from build123d import *

# Parameters (mm, degrees)
SKETCH1_W           = 4.6
SKETCH1_H           = 2.55
BOSS_EXTRUDE1_DEPTH = 4.6
SKETCH2_W           = 7.97
SKETCH2_H           = 2.55
BOSS_EXTRUDE2_DEPTH = 6.22
SKETCH3_W           = 4.6
SKETCH3_H           = 0.85
BOSS_EXTRUDE3_DEPTH = 0.17
SKETCH4_W           = 4.8
SKETCH4_H           = 2.55
CUT_EXTRUDE1_DEPTH  = 1.29
SKETCH5_W           = 6.77
SKETCH5_H           = 1.15
CUT_EXTRUDE2_DEPTH  = 5.3
CUT_EXTRUDE3_REACH  = 4.55
SKETCH7_W           = 1
SKETCH7_H           = 0.35
BOSS_EXTRUDE4_DEPTH = 3.3
SKETCH8_R           = 0.75
BOSS_EXTRUDE5_DEPTH = 3
SKETCH9_R           = 0.3
BOSS_EXTRUDE6_DEPTH = 1


with BuildPart() as part:
    # Sketch1 → Boss-Extrude1 (new body)
    with BuildSketch(Plane.XY):
        Rectangle(SKETCH1_W, SKETCH1_H)
    extrude(amount=BOSS_EXTRUDE1_DEPTH)

    # Sketch2 → Boss-Extrude2 (add)
    with BuildSketch(Plane.XY.offset(4.6)):
        Rectangle(SKETCH2_W, SKETCH2_H)
    extrude(amount=BOSS_EXTRUDE2_DEPTH)

    # Sketch3 → Boss-Extrude3 (add)
    with BuildSketch(Plane(origin=(0, 1.275, 0), x_dir=(1, 0, 0), z_dir=(0, 1, 0))):
        with Locations((0, -0.425)):
            Rectangle(SKETCH3_W, SKETCH3_H)
    extrude(amount=BOSS_EXTRUDE3_DEPTH)

    # Sketch4 → Cut-Extrude1 (cut)
    with BuildSketch(Plane.XY.offset(10.82)):
        Rectangle(SKETCH4_W, SKETCH4_H)
    extrude(amount=-CUT_EXTRUDE1_DEPTH, mode=Mode.SUBTRACT)

    # Sketch5 → Cut-Extrude2 (cut)
    with BuildSketch(Plane.XY.offset(10.82)):
        with Locations((0, -0.2)):
            Rectangle(SKETCH5_W, SKETCH5_H)
    extrude(amount=-CUT_EXTRUDE2_DEPTH, mode=Mode.SUBTRACT)

    # Sketch6 → Cut-Extrude3 (cut, up to next)
    with BuildSketch(Plane(origin=(0, 1.275, 0), x_dir=(1, 0, 0), z_dir=(0, 1, 0)), mode=Mode.PRIVATE) as cut_extrude3_sk1:
        Polygon((2.3, -8.515925997), (2.3, -5.52), (-2.3, -5.52), (-2.3, -8.515925997), (-2.3, -9.53), (2.3, -9.53), align=None)
    cut_extrude3_tool1 = extrude(cut_extrude3_sk1.sketch, amount=-CUT_EXTRUDE3_REACH, mode=Mode.PRIVATE) & part.part
    add(cut_extrude3_tool1.solids().sort_by_distance((0, 1.275, 7.525))[0], mode=Mode.SUBTRACT)
    # Sketch6 → Cut-Extrude3 (cut, up to next)
    with BuildSketch(Plane(origin=(0, 1.275, 0), x_dir=(1, 0, 0), z_dir=(0, 1, 0)), mode=Mode.PRIVATE) as cut_extrude3_sk2:
        Polygon((-2.3, -9.53), (-2.3, -8.515925997), (-2.6, -8.944370399), (-2.6, -9.244370399), (-2.4, -9.53), align=None)
    cut_extrude3_tool2 = extrude(cut_extrude3_sk2.sketch, amount=-CUT_EXTRUDE3_REACH, mode=Mode.PRIVATE) & part.part
    add(cut_extrude3_tool2.solids().sort_by_distance((-2.423539, 1.275, 9.078047))[0], mode=Mode.SUBTRACT)
    # Sketch6 → Cut-Extrude3 (cut, up to next)
    with BuildSketch(Plane(origin=(0, 1.275, 0), x_dir=(1, 0, 0), z_dir=(0, 1, 0)), mode=Mode.PRIVATE) as cut_extrude3_sk3:
        Polygon((2.6, -8.944370399), (2.3, -8.515925997), (2.3, -9.53), (2.4, -9.53), (2.6, -9.244370399), align=None)
    cut_extrude3_tool3 = extrude(cut_extrude3_sk3.sketch, amount=-CUT_EXTRUDE3_REACH, mode=Mode.PRIVATE) & part.part
    add(cut_extrude3_tool3.solids().sort_by_distance((2.423539, 1.275, 9.078047))[0], mode=Mode.SUBTRACT)

    # Sketch7 → Boss-Extrude4 (add)
    with BuildSketch(Plane.XY.offset(5.52)):
        with Locations((1, 0)):
            Rectangle(SKETCH7_W, SKETCH7_H)
        with Locations((-1, 0)):
            Rectangle(SKETCH7_W, SKETCH7_H)
    extrude(amount=BOSS_EXTRUDE4_DEPTH)

    # Sketch8 → Boss-Extrude5 (add)
    with BuildSketch(Plane(origin=(0, 0, 0), x_dir=(-1, 0, 0), z_dir=(0, 0, -1))):
        with Locations((-1, 0)):
            Circle(SKETCH8_R)
        with Locations((1, 0)):
            Circle(SKETCH8_R)
    extrude(amount=BOSS_EXTRUDE5_DEPTH)

    # Sketch9 → Boss-Extrude6 (add)
    with BuildSketch(Plane(origin=(0, 0, -3), x_dir=(-1, 0, 0), z_dir=(0, 0, -1))):
        with Locations((-1, 0)):
            Circle(SKETCH9_R)
        with Locations((1, 0)):
            Circle(SKETCH9_R)
    extrude(amount=BOSS_EXTRUDE6_DEPTH)


solid = part.part
Work out the finished part from the listing and answer in its coordinate system (mm). A direction names the side the tool comes from. Round coordinates to 2 decimals unless told otherwise and drop trailing zeros. Write each loop counter-clockwise with the first axis right and the second up, starting at its lowest first coordinate (ties: lowest second). Pieces come first, ordered by that corner, then holes. Notation, with made-up numbers: (48.25, -34) -> (66.25, -34) arc R25 cw to (66.25, -7) -> close; hole circle Ø10 at (-10, 87). An arc over 180 degrees is marked (long way). Write each question's results on one line, items separated by ' | '.
Item 1: Find the intervals of material crossed by line 1 along X through (y, z) = (0, 8.25) (3 decimals); line 2 along X through (y, z) = (-0.1, 10) (3 decimals); line 3 along X through (y, z) = (-0.95, 10) (3 decimals), in increasing order. Write a range as [from, to].
Result set:
line 1: [-3.985, -3.385], [-1.5, -0.5], [0.5, 1.5], [3.385, 3.985] | line 2: [-3.985, -3.385], [3.385, 3.985] | line 3: [-3.985, -2.4], [2.4, 3.985]
Item 2: A cutting plane is placed at A-A, the plane z = 6.25. Determine the outline of the cut face in (x, y) (3 decimals).
Result set:
outline: (-3.985, -1.275) -> (3.985, -1.275) -> (3.985, 1.275) -> (2.3, 1.275) -> (2.3, 0.375) -> (3.385, 0.375) -> (3.385, -0.775) -> (-3.385, -0.775) -> (-3.385, 0.375) -> (-2.3, 0.375) -> (-2.3, 1.275) -> (-3.985, 1.275) -> close; (-1.5, -0.175) -> (-0.5, -0.175) -> (-0.5, 0.175) -> (-1.5, 0.175) -> close; (0.5, -0.175) -> (1.5, -0.175) -> (1.5, 0.175) -> (0.5, 0.175) -> close
Item 3: A cutting plane is placed at B-B, the plane y = -0.6. Determine the outline of the cut face in (x, z) (3 decimals), plus the area to 3 significant figures.
Result set:
outline: (-3.985, 4.6) -> (-2.3, 4.6) -> (-2.3, 0) -> (-1.45, 0) -> (-1.45, -3) -> (-0.55, -3) -> (-0.55, 0) -> (0.55, 0) -> (0.55, -3) -> (1.45, -3) -> (1.45, 0) -> (2.3, 0) -> (2.3, 4.6) -> (3.985, 4.6) -> (3.985, 10.82) -> (3.385, 10.82) -> (3.385, 5.52) -> (-3.385, 5.52) -> (-3.385, 10.82) -> (-3.985, 10.82) -> close | area: 40.3 mm^2
Item 4: A cutting plane is placed at D-D, the plane z = 2.5. Determine the outline of the cut face in (x, y) (3 decimals), plus the area to 3 significant figures.
Result set:
outline: (-2.3, -1.275) -> (2.3, -1.275) -> (2.3, 1.275) -> (-2.3, 1.275) -> close | area: 11.7 mm^2
Item 5: A cutting plane is placed at C-C, the plane x = 1. Determine the outline of the cut face in (y, z) (3 decimals), plus the area to 3 significant figures.
Result set:
outline: (-1.275, 0) -> (-0.75, 0) -> (-0.75, -3) -> (-0.3, -3) -> (-0.3, -4) -> (0.3, -4) -> (0.3, -3) -> (0.75, -3) -> (0.75, 0) -> (1.445, 0) -> (1.445, 0.85) -> (1.275, 0.85) -> (1.275, 5.52) -> (0.175, 5.52) -> (0.175, 8.82) -> (-0.175, 8.82) -> (-0.175, 5.52) -> (-0.775, 5.52) -> (-0.775, 9.53) -> (-1.275, 9.53) -> close | area: 22.5 mm^2
Item 6: Which of the six approach directions +Z, -Z, +X, -X, +Y, -Y give full straight-line access (tool end or side, diameter ignored) to faces 5 (the face through (-2.3, 0, 2)), 6 (the face through (0, 1.275, 5)), 7 (the face through (-3.385, 0, 8))?
Result set:
face 5: -Z, -X, +Y, -Y | face 6: +Z, +X, -X, +Y | face 7: +Z
Item 7: The mould has two halves that part along X. Classify faces 1 (the face through (0.285, 0.225, -1.479)), 2 (the face through (3, 0.375, 8)), 3 (the face through (2.3, 0, 2)), 4 (the face through (0, -1.275, 5)): +X half, -X half, draft (parallel to the pull), parting line (faces both ways), or undercut.
Result set:
face 1: undercut | face 2: undercut | face 3: +X half | face 4: draft
Item 8: Flat-ended cylindrical pins translate along their axes: P1, Ø1.5, axis at x = 0, y = 0.5, coming from the -Z side; P2, Ø0.8, axis at y = 0.5, z = 3.5, coming from the +X side. Find the tip coordinate at first contact, or state that the pin passes through.
Result set:
P1: z = -3 | P2: x = 2.3
